Geometry check sheet. Reference: drawing and pictorial views, mm from the part's lowest x, y, z. Give positions to 0.01 mm unless a question says otherwise; leave off trailing zeros. Write each loop counter-clockwise with the first axis right and the second up, starting at its lowest first coordinate (ties: lowest second). Pieces come first, ordered by that corner, then holes. Notation, with made-up numbers: (-39.75, -31.75) -> (-6.75, -31.75) arc R21 ccw to (-6.75, -21.75) -> close; hole circle Ø5 at (89, 42.25). An arc over 180 degrees is marked (long way). Use a Markdown table: item, result. Add a question column.
1. Cross-section at B-B (y = 28.78). Enter the section's corners in (x, z), then the cut area to 3 significant figures.
2. Cross-section at D-D (y = 64.5). Enter the section's corners in (x, z).
3. Scan lines: probe 1 along X at (y, z) = (64.5, 1.3); probe 2 along Y at (x, z) = (11, 2.4); probe 3 along X at (y, z) = (33, 2.05). Record each from-to range of solid material in increasing order. Write a range as [from, to].
4. Cross-section at A-A (x = 21). Enter the section's corners in (y, z), then the cut area to 3 significant figures.
5. Cross-section at C-C (z = 2.25). Enter the section's corners in (x, y).
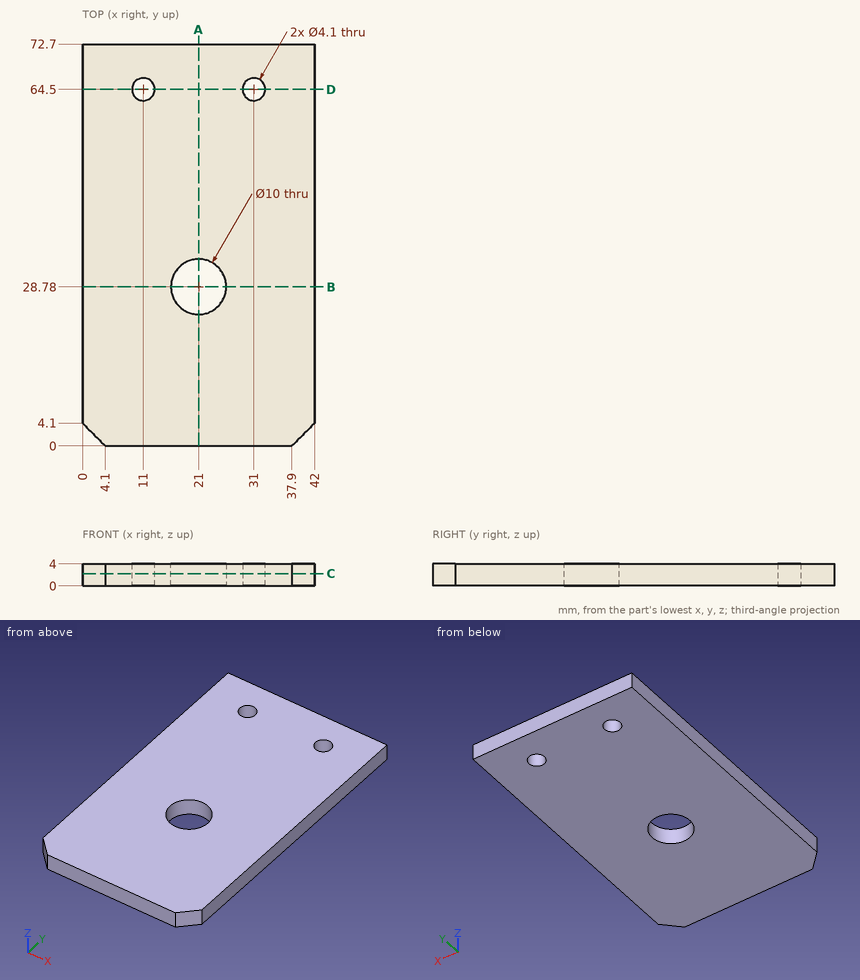
Worked answers:
| question | item | result |
|---|---|---|
| 1 | outline | (0, 0) -> (16, 0) -> (16, 4) -> (0, 4) -> close; (26, 0) -> (42, 0) -> (42, 4) -> (26, 4) -> close |
| 1 | area | 128 mm² |
| 2 | outline | (0, 0) -> (8.95, 0) -> (8.95, 4) -> (0, 4) -> close; (13.05, 0) -> (28.95, 0) -> (28.95, 4) -> (13.05, 4) -> close; (33.05, 0) -> (42, 0) -> (42, 4) -> (33.05, 4) -> close |
| 3 | probe 1 | x = [0, 8.95], [13.05, 28.95], [33.05, 42] |
| 3 | probe 2 | y = [0, 62.45], [66.55, 72.7] |
| 3 | probe 3 | x = [0, 18.32], [23.68, 42] |
| 4 | outline | (0, 0) -> (23.78, 0) -> (23.78, 4) -> (0, 4) -> close; (33.78, 0) -> (72.7, 0) -> (72.7, 4) -> (33.78, 4) -> close |
| 4 | area | 251 mm² |
| 5 | outline | (0, 4.1) -> (4.1, 0) -> (37.9, 0) -> (42, 4.1) -> (42, 72.7) -> (0, 72.7) -> close; hole circle Ø4.1 at (11, 64.5); hole circle Ø10 at (21, 28.78); hole circle Ø4.1 at (31, 64.5) |
